Could you check a few things on this drawing? It's one solid part, dimensions in mm from its lowest x, y, z. A direction names the side the tool comes from. Give positions to 0.01 mm unless a question says otherwise; leave off trailing zeros. Loops run counter-clockwise (first coordinate to the right, second up) from the corner with the lowest first, then second, coordinate; pieces in that order, holes last. Notation, with made-up numbers: (-17, 65) - (16, 65) arc R14 cw to (16, 86) - close; hole circle Ø8 at (2, -2). An arc over 180 degrees is marked (long way). Return JSON: item names as keys, results as strings. Group by question number.
(1) If we section it at D-D (x = 25): Please give me the cut outline in (y, z).
(2) For P1, Ø5, axis at x = 30, z = 3, coming from the -Y side; P2, Ø5, axis at x = 9, z = 3, coming from the +Y side; P3, Ø2.5, axis at x = 32, y = 11.5, coming from the +Z side; P4, Ø1, axis at x = 11, y = 18, coming from the -Z side, each with a flat end and sliding along its axis, tell me the tip position at first contact or that it passes through.
(3) I need wall thicknesses on probe 1 along X at (y, z) = (1.9, 3); probe 2 along X at (y, z) = (12.5, 8.25); probe 3 along Z at (x, y) = (8, 12.5). Which ranges of each line are inside material? Lowest first, please. Write a range as [from, to].
(4) If we section it at C-C (z = 8.75): Please give me the cut outline in (x, y).
(5) If we section it at A-A (x = 30): Please give me the cut outline in (y, z), then the cut area to 3 significant figures.
(6) If we section it at B-B (z = 3): Please give me the cut outline in (x, y), then the cut area to 3 significant figures.
(7) If we mould it in two halves opening along Z, with no side actions, what happens to the marked faces 3, 4 and 5? For each: released by +Z, released by -Z, zero draft, split by the parting line, or undercut.
(8) On a 3-axis mill with a long thin cutter (end or side, diameter ignored), from which of +Z, -Z, +X, -X, +Y, -Y can I reach the whole of each face in a straight line? I mean the marked faces 1 and 2. Say none if no direction works.
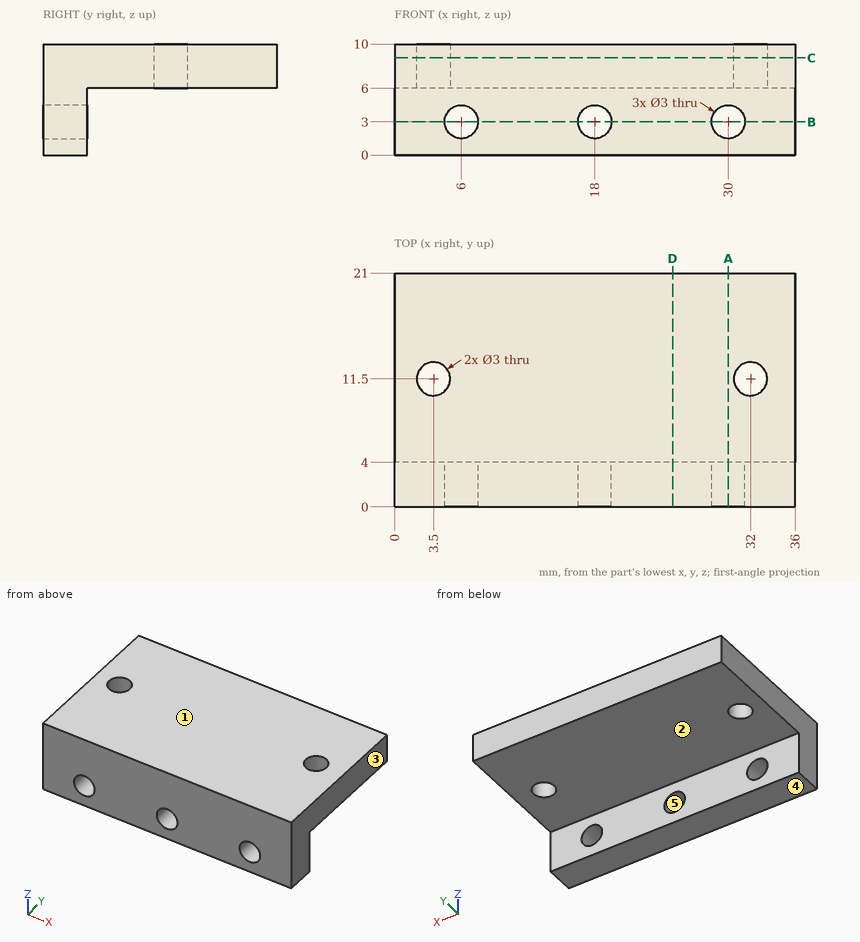
Values:
{
 "1": {"outline": "(0, 0) - (4, 0) - (4, 6) - (21, 6) - (21, 10) - (0, 10) - close"},
 "2": {"P1": "y = 0", "P2": "y = 4", "P3": "through", "P4": "z = 6"},
 "3": {"probe 1": "[0, 4.5], [7.5, 16.5], [19.5, 28.5], [31.5, 36]", "probe 2": "[0, 2.38], [4.62, 30.88], [33.12, 36]", "probe 3": "[6, 10]"},
 "4": {"outline": "(0, 0) - (36, 0) - (36, 21) - (0, 21) - close; hole circle Ø3 at (3.5, 11.5); hole circle Ø3 at (32, 11.5)"},
 "5": {"outline": "(0, 0) - (4, 0) - (4, 1.5) - (0, 1.5) - close; (0, 4.5) - (4, 4.5) - (4, 6) - (21, 6) - (21, 10) - (0, 10) - close", "area": "96.0 mm2"},
 "6": {"outline": "(0, 0) - (4.5, 0) - (4.5, 4) - (0, 4) - close; (7.5, 0) - (16.5, 0) - (16.5, 4) - (7.5, 4) - close; (19.5, 0) - (28.5, 0) - (28.5, 4) - (19.5, 4) - close; (31.5, 0) - (36, 0) - (36, 4) - (31.5, 4) - close", "area": "108 mm2"},
 "7": {"face 3": "zero draft", "face 4": "released by -Z", "face 5": "undercut"},
 "8": {"face 1": "+Z, +X, -X, +Y, -Y", "face 2": "-Z, +X, -X, +Y"}
}
